Can you work these out from the drawing? Everything is in mm from the part's minimum corner. Give positions to 0.01 mm unless a question says otherwise; leave off trailing zeros. Order: outer loops, then holes, each group sorted by start corner. A loop starts at its lowest first (then second) coordinate and runs counter-clockwise, first axis right, second up. Notation, with made-up numbers: (73.25, 72) -> (102.25, 72) arc R23 cw to (102.25, 83) -> close; hole circle Ø3 at (23, 19.5). An arc over 180 degrees is marked (long way). One line per item, written item: value.
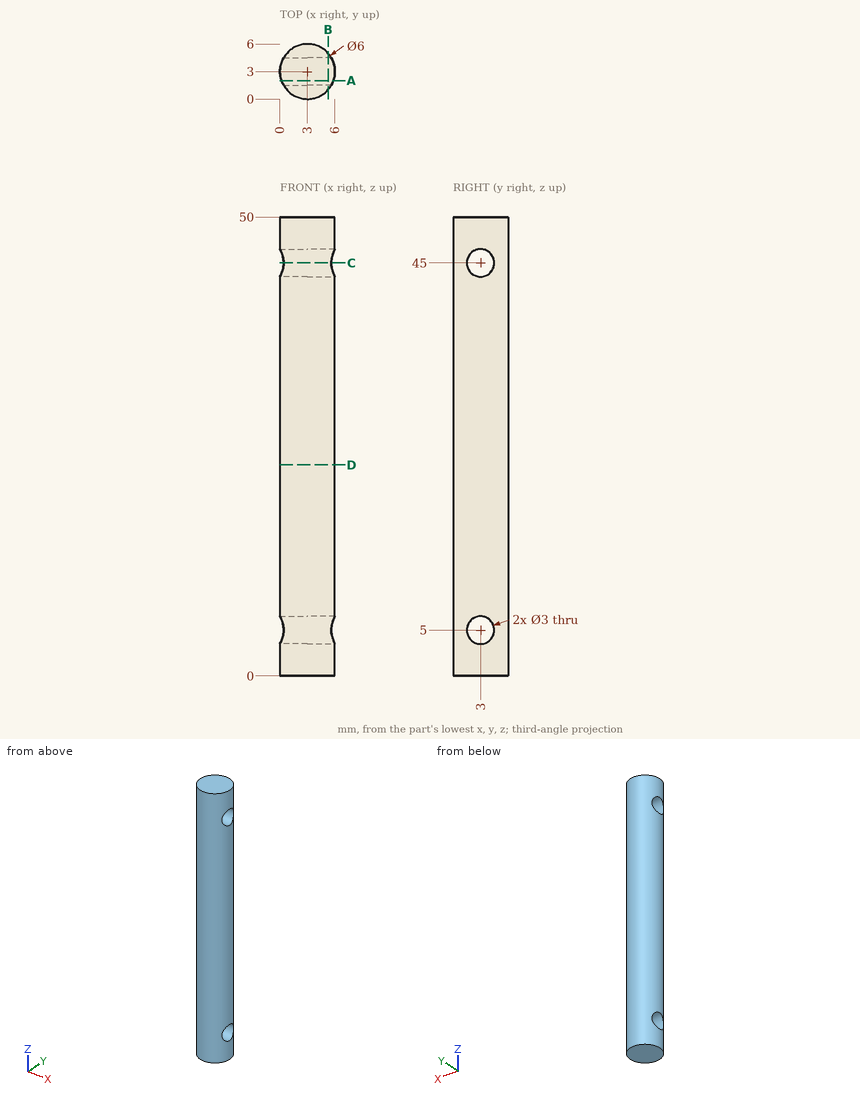
1) Suppose I cut it at B-B, the plane x = 5.25. Write out the boundary of the cut face in (y, z), then the cut area to 3 significant figures.
Answer below:
outline: (1.02, 0) -> (4.98, 0) -> (4.98, 50) -> (1.02, 50) -> close; hole circle Ø3 at (3, 5); hole circle Ø3 at (3, 45)
area: 184 mm2
2) Suppose I cut it at C-C, the plane z = 45. Write out the boundary of the cut face in (x, y), then the cut area to 3 significant figures.
Answer below:
outline: (0.4, 1.5) arc R3 ccw to (5.6, 1.5) -> close; (0.4, 4.5) -> (5.6, 4.5) arc R3 ccw to start
area: 11.1 mm2
3) Suppose I cut it at A-A, the plane y = 2. Write out the boundary of the cut face in (x, z).
Answer below:
outline: (0.17, 0) -> (5.83, 0) -> (5.83, 3.88) -> (0.17, 3.88) -> close; (0.17, 6.12) -> (5.83, 6.12) -> (5.83, 43.88) -> (0.17, 43.88) -> close; (0.17, 46.12) -> (5.83, 46.12) -> (5.83, 50) -> (0.17, 50) -> close
4) Suppose I cut it at D-D, the plane z = 23. Write out the boundary of the cut face in (x, y), then the cut area to 3 significant figures.
Answer below:
outline: circle Ø6 at (3, 3)
area: 28.3 mm2
5) If I drill on line 1 along Z through (x, y) = (2.75, 3.5); line 2 along Z through (x, y) = (4, 2); line 3 along X through (y, z) = (3.25, 21.5), over which ranges is the centre line in solid material (lowest first)?
Answer below:
line 1: z = 0 to 3.59, 6.41 to 43.59, 46.41 to 50
line 2: z = 0 to 3.88, 6.12 to 43.88, 46.12 to 50
line 3: x = 0.01 to 5.99
6) For P1, Ø2, axis at y = 1, z = 12, coming from the +X side; P2, Ø1, axis at y = 4, z = 38.5, coming from the +X side; P3, Ø1, axis at x = 1, z = 23.5, coming from the -Y side, each with a flat end and sliding along its axis, tell me the tip position at first contact or that it passes through.
Answer below:
P1: stops at x = 5.83
P2: stops at x = 5.96
P3: stops at y = 0.4
